Check sheet for the drawn part. Datum: minimum x, y, z corner. Units: mm. Coordinates: 2 decimals unless noted, no trailing zeros. Write each loop counter-clockwise with the first axis right and the second up, starting at its lowest first coordinate (ties: lowest second). Pieces come first, ordered by that corner, then holes. Notation, with made-up numbers: M 4.5,-20 L 43.5,-20 A28 cw 43.5,9 Z; hole C 84,-40 d4. An arc over 180 degrees is marked long. Answer as CSV lines item,"result".
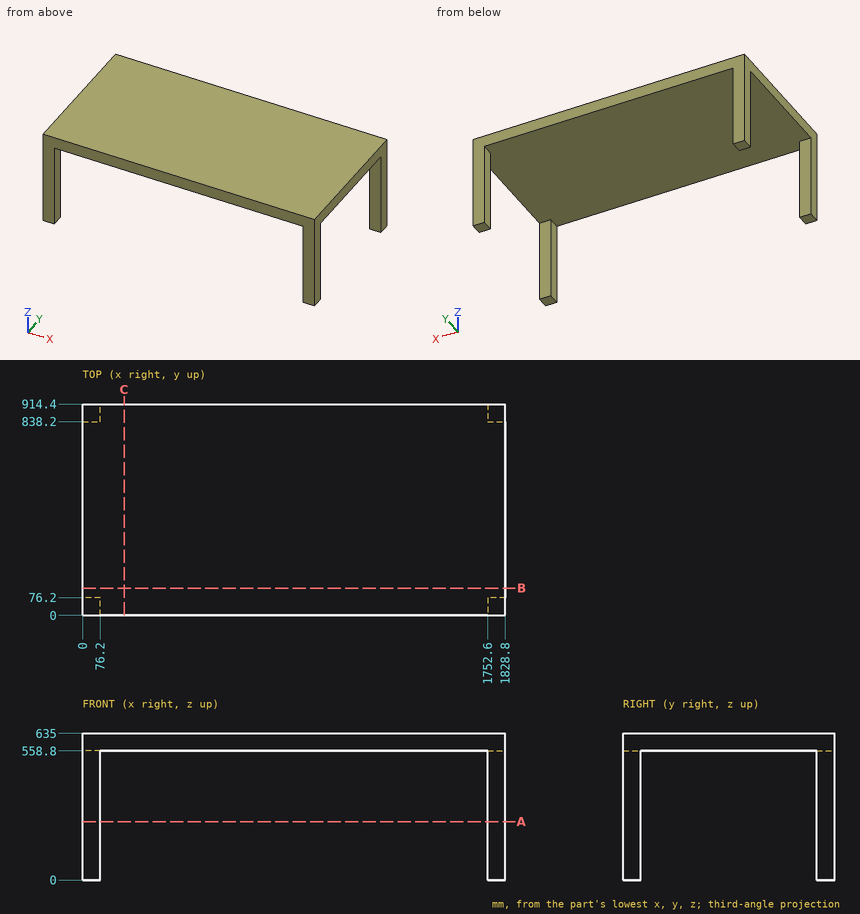
1) Section check A-A, the plane z = 253. Record the boundary of the cut face in (x, y), plus the area to 3 significant figures.
Answer key:
outline,"M 0,0 L 76.2,0 L 76.2,76.2 L 0,76.2 Z; M 0,838.2 L 76.2,838.2 L 76.2,914.4 L 0,914.4 Z; M 1752.6,0 L 1828.8,0 L 1828.8,76.2 L 1752.6,76.2 Z; M 1752.6,838.2 L 1828.8,838.2 L 1828.8,914.4 L 1752.6,914.4 Z"
area,"23,200 mm2"
2) Section check B-B, the plane y = 117.5. Record the boundary of the cut face in (x, z), plus the area to 3 significant figures.
Answer key:
outline,"M 0,558.8 L 1828.8,558.8 L 1828.8,635 L 0,635 Z"
area,"139,000 mm2"
3) Thickness scan on line 1 along X through (y, z) = (53.5, 274.5); line 2 along Z through (x, y) = (563.5, 606). Record the ranges inside material, lowest first.
Answer key:
line 1,"x = 0 to 76.2, 1752.6 to 1828.8"
line 2,"z = 558.8 to 635"
4) Depth check by flat-ended pin: P1, Ø5, axis at x = 542.5, y = 151, coming from the -Z side. Enter the tip coordinate at first touch or a pass-through.
Answer key:
P1,"stops at z = 558.8"
5) Section check C-C, the plane x = 180.5. Record the boundary of the cut face in (y, z), plus the area to 3 significant figures.
Answer key:
outline,"M 0,558.8 L 914.4,558.8 L 914.4,635 L 0,635 Z"
area,"69,700 mm2"
